Can you work these out from the drawing? Everything is in mm from the part's minimum corner. Round coordinates to 2 decimals unless told otherwise and drop trailing zeros. Loops run counter-clockwise (first coordinate to the right, second up) from the corner with the lowest first, then second, coordinate; pieces in that order, holes last. Notation, with made-up numbers: (3.25, -25.75) -> (39.25, -25.75) arc R9 cw to (39.25, -11.75) -> close; hole circle Ø11 at (-19, -19). An arc over 180 degrees is marked (long way). One line per item, written item: value.
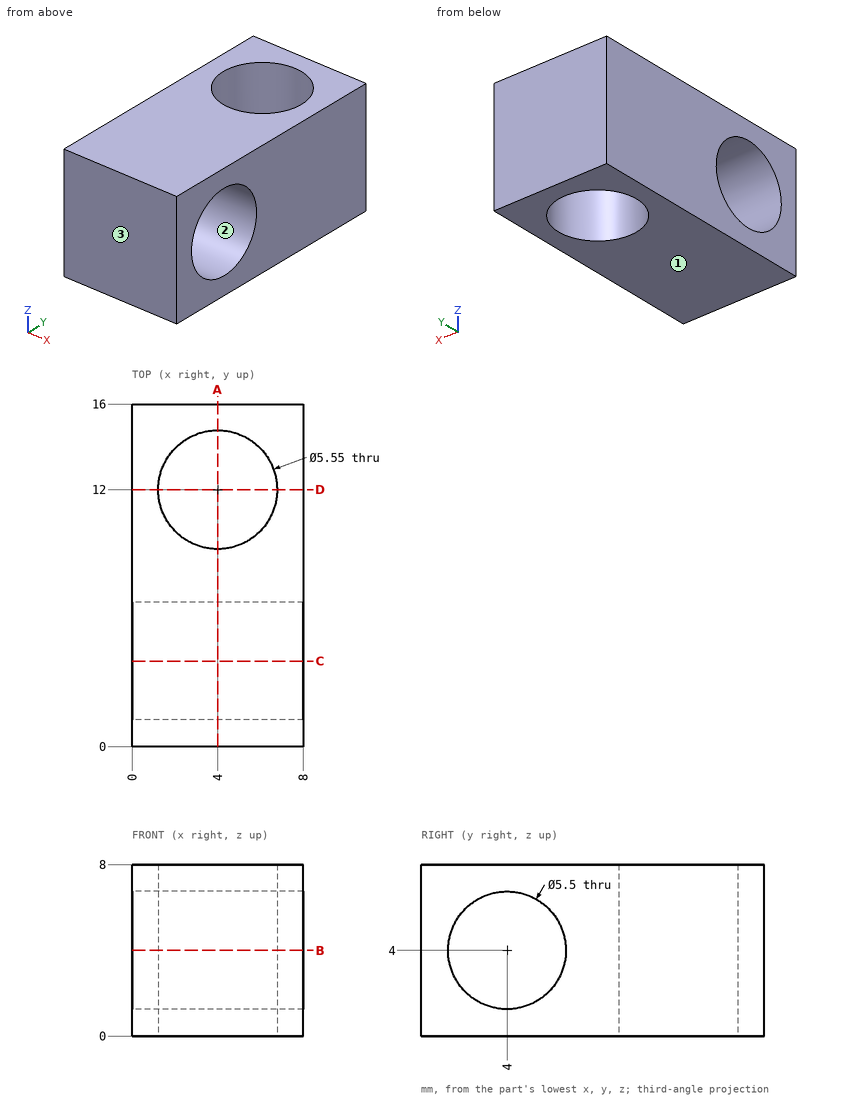
(1) Imagine slicing it at A-A on x = 4. Write out the boundary of the cut face in (y, z) (3 decimals), then the cut area to 3 significant figures.
Results below:
outline: (0, 0) -> (9.225, 0) -> (9.225, 8) -> (0, 8) -> close; (14.775, 0) -> (16, 0) -> (16, 8) -> (14.775, 8) -> close; hole circle Ø5.5 at (4, 4)
area: 59.8 mm²
(2) Imagine slicing it at D-D on y = 12. Write out the boundary of the cut face in (x, z) (3 decimals), then the cut area to 3 significant figures.
Results below:
outline: (0, 0) -> (1.225, 0) -> (1.225, 8) -> (0, 8) -> close; (6.775, 0) -> (8, 0) -> (8, 8) -> (6.775, 8) -> close
area: 19.6 mm²
(3) Imagine slicing it at C-C on y = 4. Write out the boundary of the cut face in (x, z).
Results below:
outline: (0, 0) -> (8, 0) -> (8, 1.25) -> (0, 1.25) -> close; (0, 6.75) -> (8, 6.75) -> (8, 8) -> (0, 8) -> close
(4) Imagine slicing it at B-B on z = 4. Write out the boundary of the cut face in (x, y) (3 decimals), then the cut area to 3 significant figures.
Results below:
outline: (0, 0) -> (8, 0) -> (8, 1.25) -> (0, 1.25) -> close; (0, 6.75) -> (8, 6.75) -> (8, 16) -> (0, 16) -> close; hole circle Ø5.55 at (4, 12)
area: 59.8 mm²
(5) For pin 1 Ø4.5 at (y, z) = (4, 4) entering from +X, with a flat end and sliding along its axis, tell me the tip position at first contact or that it passes through.
Results below:
pin 1: passes through
(6) We'd pull the mould along Z, two halves only. Please class the marked faces 1, 2 and 3: +Z half, -Z half, draft (parallel to the pull), parting line (faces both ways), or undercut.
Results below:
face 1: -Z half
face 2: undercut
face 3: draft
(7) Please list where these lines run through material, in increasing order: L1, parallel to Y at x = 4, z = 0.5 (3 decimals); L2, parallel to Y at x = 4.75, z = 5.5; L3, parallel to Z at x = 5.5, y = 4.
Results below:
L1: y = 0 to 9.225, 14.775 to 16
L2: y = 0 to 1.7, 6.3 to 9.33, 14.67 to 16
L3: z = 0 to 1.25, 6.75 to 8
